CAD build for the part. Positions are in the model's coordinates, mm. A direction names the side the tool comes from. Give positions to 0.01 mm unless a question says otherwise; leave off trailing zeros. Order: outer loops, then holes, each group sorted by start corner. A loop starts at its lowest first (then second) coordinate and runs counter-clockwise, first axis right, second up. Notation, with made-up numbers: M 46,-39 L 91,-39 A6 ccw 91,-35 Z; hole C 66.5,-9.5 d7. An arc over 180 degrees is marked long. Put each result on its own line as item: value. Start each with the question number.
1) Pin check, flat tips, straight feed: pin 1 (2 mm diameter, centred on x = 7, y = 31, fed in from +Z); pin 2 (5.5 mm diameter, centred on x = 7.5, y = 30, fed in from -Z); pin 3 (10 mm diameter, centred on x = -25, z = 38, fed in from +Y); pin 4 (1.5 mm diameter, centred on x = -17, y = 4.5, fed in from -Z). Stop position of each tip, or through.
2) Drill centre lines: line 1 (X direction, y = 30, z = 7.4); line 2 (Y direction, x = -20, z = 43); line 3 (Z direction, x = -5, y = 33.5). Where is each one in solid material? Low to high. Write a range as [from, to].
3) Two-plate mould, pull along Z, no slides. Class faces 5 (the face through (13.045, -2.465, 44.926)), 6 (the face through (0, 15, 0)), 7 (the face through (-15, 3, 5)), 8 (the face through (-44.45, -0.07, 65.293)): released by +Z, released by -Z, zero draft, split by the parting line, or undercut.
4) Cut at A-A (y = 30). Write the cut outline in (x, z), and give its area (3 significant figures).
5) Tool access for faces 1 (the face through (7.04, 33.47, 6.82)), 2 (the face through (14, 23, 6)), 3 (the face through (-14, 22, 6)), 4 (the face through (-3, 0, 36)): list every direction of +Z, -Z, +X, -X, +Y, -Y with a clear straight run to the whole face (end or side of a thin tool).
6) Cut at B-B (y = 23). Write the cut outline in (x, z).
7) Cut at C-C (y = 3). Give the number of separate pieces and of enclosed holes in the cut face, and give its area (3 significant figures).
```python
from build123d import *

# Parameters (mm, degrees)
CROQUIS1_R                                           = 3
SALIENTE_EXTRUIR1_DEPTH                              = 5
CROQUIS2_W                                           = 30
CROQUIS2_H                                           = 30
SALIENTE_EXTRUIR2_DEPTH                              = 8
REFRENTADO_PARA_TORNILLO_CON_CABEZA_TRON_D           = 3.4
REFRENTADO_PARA_TORNILLO_CON_CABEZA_TRON_CBORE_D     = 7
REFRENTADO_PARA_TORNILLO_CON_CABEZA_TRON_CBORE_DEPTH = 2.4
CROQUIS11_R                                          = 6.5
CORTAR_EXTRUIR3_DEPTH                                = 5
REDONDEO8_R                                          = 5


with BuildPart() as part:
    # Croquis1 → Saliente-Extruir1 (new, symmetric)
    with BuildSketch(Plane(origin=(0, 0, 0), x_dir=(-1, 0, 0), z_dir=(0, 1, 0))):
        with BuildLine():
            Line((15, 0), (-15, 0))
            Line((-15, 0), (-15, 37.5217))
            ThreePointArc((-15, 37.5217), (-12.990381057, 45.0217), (-7.5, 50.512081057))
            Line((-7.5, 50.512081057), (35.801270189, 75.512081057))
            ThreePointArc((35.801270189, 75.512081057), (56.291651246, 70.0217), (50.801270189, 49.531318943))
            Line((50.801270189, 49.531318943), (15, 28.861445962))
            Line((15, 28.861445962), (15, 0))
        make_face()
        with Locations(Location((0, 37.5217, 0), (0, 0, 90))):
            Circle(CROQUIS1_R, mode=Mode.SUBTRACT)
        with Locations(Location((43.301270189, 62.5217, 0), (0, 0, 90))):
            Circle(CROQUIS1_R, mode=Mode.SUBTRACT)
    extrude(amount=SALIENTE_EXTRUIR1_DEPTH, both=True)

    # Croquis2 → Saliente-Extruir2 (add)
    with BuildSketch(Plane(origin=(0, 0, 0), x_dir=(1, 0, 0), z_dir=(0, 0, -1))):
        with Locations((0, -20)):
            Rectangle(CROQUIS2_W, CROQUIS2_H)
    extrude(amount=-SALIENTE_EXTRUIR2_DEPTH)

    # Refrentado para tornillo con cabeza troncocónica de M31 (through all)
    with Locations(Plane.XY.offset(8)):
        with Locations((-7.5, 30), (7.5, 30)):
            CounterBoreHole(REFRENTADO_PARA_TORNILLO_CON_CABEZA_TRON_D / 2, REFRENTADO_PARA_TORNILLO_CON_CABEZA_TRON_CBORE_D / 2, REFRENTADO_PARA_TORNILLO_CON_CABEZA_TRON_CBORE_DEPTH)

    # Croquis11 → Cortar-Extruir3 (cut)
    with BuildSketch(Plane.XZ.offset(5)):
        with Locations(Location((0, 37.5217, 0), (0, 0, 270))):
            Circle(CROQUIS11_R)
    extrude(amount=-CORTAR_EXTRUIR3_DEPTH, mode=Mode.SUBTRACT)

    # Redondeo8
    # the kernel refuses this fillet: 5 mm, written as the material it adds along each edge
    with BuildSketch(Plane(origin=(15, 5, 8), x_dir=(0, 0, 1), z_dir=(-1, 0, 0))) as redondeo8_piece_1:
        with BuildLine():
            CenterArc((REDONDEO8_R, REDONDEO8_R), REDONDEO8_R, 180, 90)
            Line((0, REDONDEO8_R), (0, 0))
            Line((0, 0), (REDONDEO8_R, 0))
        make_face()
    extrude(amount=30)
    # the kernel refuses this fillet: 5 mm, written as the material it takes off along each edge
    with BuildSketch(Plane(origin=(-50.801270189, 5, 49.531318943), x_dir=(0.4999999999999951, 0, 0.8660254037844415), z_dir=(0.8660254037844415, 0, -0.49999999999999517))) as redondeo8_2_piece_1_section:
        with BuildLine():
            CenterArc((REDONDEO8_R, REDONDEO8_R), REDONDEO8_R, 180, 90)
            Line((0, REDONDEO8_R), (0, 0))
            Line((0, 0), (REDONDEO8_R, 0))
        make_face()
    redondeo8_2_piece_1 = extrude(amount=53.839745962, mode=Mode.PRIVATE)
    redondeo8_2_piece_1 = split(redondeo8_2_piece_1, bisect_by=Plane(origin=(-15, 3.85828394, 40.323429829), z_dir=(-1, 0, 0)), keep=Keep.TOP, mode=Mode.PRIVATE)
    add(redondeo8_2_piece_1, mode=Mode.SUBTRACT)
    with BuildSketch(Plane(origin=(-43.301270189, 5, 62.5217), x_dir=(0.4999999999999953, 0, 0.8660254037844414), z_dir=(0.8660254037844414, 0, -0.4999999999999953))) as redondeo8_2_piece_2:
        with BuildLine():
            CenterArc((15 - REDONDEO8_R, REDONDEO8_R), REDONDEO8_R, 270, 90)
            Line((15, REDONDEO8_R), (15, 0))
            Line((15, 0), (15 - REDONDEO8_R, 0))
        make_face()
    revolve(axis=Axis((-43.301270189, 5, 62.5217), (0, -1, 0)), revolution_arc=180, mode=Mode.SUBTRACT)
    with BuildSketch(Plane(origin=(7.5, 5, 50.512081057), x_dir=(0, -1, 0), z_dir=(-0.8660254037844416, 0, 0.499999999999995))) as redondeo8_2_piece_3:
        with BuildLine():
            CenterArc((REDONDEO8_R, -REDONDEO8_R), REDONDEO8_R, 90, 90)
            Line((0, -REDONDEO8_R), (0, 0))
            Line((0, 0), (REDONDEO8_R, 0))
        make_face()
    extrude(amount=50, mode=Mode.SUBTRACT)
    with BuildSketch(Plane(origin=(0, 5, 37.5217), x_dir=(1, 0, 0), z_dir=(0, 0, -1))) as redondeo8_2_piece_4:
        with BuildLine():
            CenterArc((15 - REDONDEO8_R, REDONDEO8_R), REDONDEO8_R, 270, 90)
            Line((15 - REDONDEO8_R, 0), (15, 0))
            Line((15, 0), (15, REDONDEO8_R))
        make_face()
    revolve(axis=Axis((0, 5, 37.5217), (0, -1, 0)), revolution_arc=60, mode=Mode.SUBTRACT)
    with BuildSketch(Plane(origin=(-15, 5, 41.361445962), x_dir=(1, 0, 0), z_dir=(0, 0, -1))) as redondeo8_2_piece_5_section:
        with BuildLine():
            CenterArc((REDONDEO8_R, REDONDEO8_R), REDONDEO8_R, 180, 90)
            Line((0, REDONDEO8_R), (0, 0))
            Line((0, 0), (REDONDEO8_R, 0))
        make_face()
    redondeo8_2_piece_5 = extrude(amount=28.361445962, mode=Mode.PRIVATE)
    redondeo8_2_piece_5 = split(redondeo8_2_piece_5, bisect_by=Plane(origin=(-10.61401453, 3.841965375, 26.329196071), z_dir=(-0.49999999999999517, 0, -0.8660254037844415)), keep=Keep.TOP, mode=Mode.PRIVATE)
    add(redondeo8_2_piece_5, mode=Mode.SUBTRACT)
    with BuildSketch(Plane(origin=(15, 47.5, 8), x_dir=(0, 0, -1), z_dir=(0, -1, 0))) as redondeo8_2_piece_6:
        with BuildLine():
            CenterArc((REDONDEO8_R, -REDONDEO8_R), REDONDEO8_R, 90, 90)
            Line((0, -REDONDEO8_R), (0, 0))
            Line((0, 0), (REDONDEO8_R, 0))
        make_face()
    extrude(amount=37.5, mode=Mode.SUBTRACT)
    with BuildSketch(Plane(origin=(-15, 10, 8), x_dir=(1, 0, 0), z_dir=(0, 1, 0))) as redondeo8_2_piece_7:
        with BuildLine():
            CenterArc((REDONDEO8_R, REDONDEO8_R), REDONDEO8_R, 180, 90)
            Line((0, REDONDEO8_R), (0, 0))
            Line((0, 0), (REDONDEO8_R, 0))
        make_face()
    extrude(amount=37.5, mode=Mode.SUBTRACT)
    with BuildSketch(Plane(origin=(15, 5, 13), x_dir=(0, -1, 0), z_dir=(0, 0, 1))) as redondeo8_2_piece_8:
        with BuildLine():
            CenterArc((REDONDEO8_R, -REDONDEO8_R), REDONDEO8_R, 90, 90)
            Line((0, -REDONDEO8_R), (0, 0))
            Line((0, 0), (REDONDEO8_R, 0))
        make_face()
    extrude(amount=24.5217, mode=Mode.SUBTRACT)
    with BuildSketch(Plane(origin=(15, 10, 13), x_dir=(0, -1, 0), z_dir=(0, 0, 1))) as redondeo8_2_piece_9:
        with BuildLine():
            CenterArc((5 + REDONDEO8_R, -REDONDEO8_R), REDONDEO8_R, 90, 90)
            Line((5, -REDONDEO8_R), (5, 0))
            Line((5, 0), (5 + REDONDEO8_R, 0))
        make_face()
    revolve(axis=Axis((15, 10, 13), (1, 0, 0)), revolution_arc=90, mode=Mode.SUBTRACT)
    with BuildSketch(Plane(origin=(-15, 10, 13), x_dir=(0, -1, 0), z_dir=(0, 0, 1))) as redondeo8_2_piece_10:
        with BuildLine():
            CenterArc((5 + REDONDEO8_R, REDONDEO8_R), REDONDEO8_R, 180, 90)
            Line((5, REDONDEO8_R), (5, 0))
            Line((5, 0), (5 + REDONDEO8_R, 0))
        make_face()
    revolve(axis=Axis((-15, 10, 13), (1, 0, 0)), revolution_arc=90, mode=Mode.SUBTRACT)
    with BuildSketch(Plane(origin=(-15, 5, 41.361445962), x_dir=(1, 0, 0), z_dir=(0, 0, -1))) as redondeo8_2_piece_11a_section:
        with BuildLine():
            CenterArc((REDONDEO8_R, REDONDEO8_R), REDONDEO8_R, 180, 90)
            Line((0, REDONDEO8_R), (0, 0))
            Line((0, 0), (REDONDEO8_R, 0))
        make_face()
    redondeo8_2_piece_11a = extrude(amount=28.361445962, mode=Mode.PRIVATE)
    redondeo8_2_piece_11a = split(redondeo8_2_piece_11a, bisect_by=Plane(origin=(-16.671225656, 3.89815345, 29.826328544), z_dir=(0.49999999999999517, 0, 0.8660254037844415)), keep=Keep.TOP, mode=Mode.PRIVATE)
    with BuildSketch(Plane(origin=(-50.801270189, 5, 49.531318943), x_dir=(0.4999999999999951, 0, 0.8660254037844415), z_dir=(0.8660254037844415, 0, -0.49999999999999517))) as redondeo8_2_piece_11b_section:
        with BuildLine():
            CenterArc((REDONDEO8_R, REDONDEO8_R), REDONDEO8_R, 180, 90)
            Line((0, REDONDEO8_R), (0, 0))
            Line((0, 0), (REDONDEO8_R, 0))
        make_face()
    redondeo8_2_piece_11b = extrude(amount=53.839745962, mode=Mode.PRIVATE)
    redondeo8_2_piece_11b = split(redondeo8_2_piece_11b, bisect_by=Plane(origin=(-15, 3.89815345, 26.931680798), z_dir=(1, 0, 0)), keep=Keep.TOP, mode=Mode.PRIVATE)
    redondeo8_2_piece_11 = redondeo8_2_piece_11a & redondeo8_2_piece_11b
    add(redondeo8_2_piece_11, mode=Mode.SUBTRACT)


solid = part.part
```
Solution:
1. pin 1: z = 5.6
1. pin 2: z = 0
1. pin 3: y = 5
1. pin 4: z = 31.88
2. line 1: [-12.37, -11], [-4, 4], [11, 12.37]
2. line 2: [-5, 5]
2. line 3: [0, 8]
3. face 5: released by +Z
3. face 6: released by -Z
3. face 7: zero draft
3. face 8: undercut
4. outline: M -15,0 L -9.2,0 L -9.2,5.6 L -11,5.6 L -11,7.9 A5 ccw -15,3 Z; M -5.8,0 L 5.8,0 L 5.8,5.6 L 4,5.6 L 4,8 L -4,8 L -4,5.6 L -5.8,5.6 Z; M 9.2,0 L 15,0 L 15,3 A5 ccw 11,7.9 L 11,5.6 L 9.2,5.6 Z
4. area: 158 mm²
5. face 1: +Z
5. face 2: +Z, +X, +Y
5. face 3: +Z, -X, +Y
5. face 4: -Y
6. outline: M -15,0 L 15,0 L 15,3 A5 ccw 10,8 L -10,8 A5 ccw -15,3 Z
7. separate pieces: 1
7. enclosed holes: 2
7. area: 2,710 mm²
